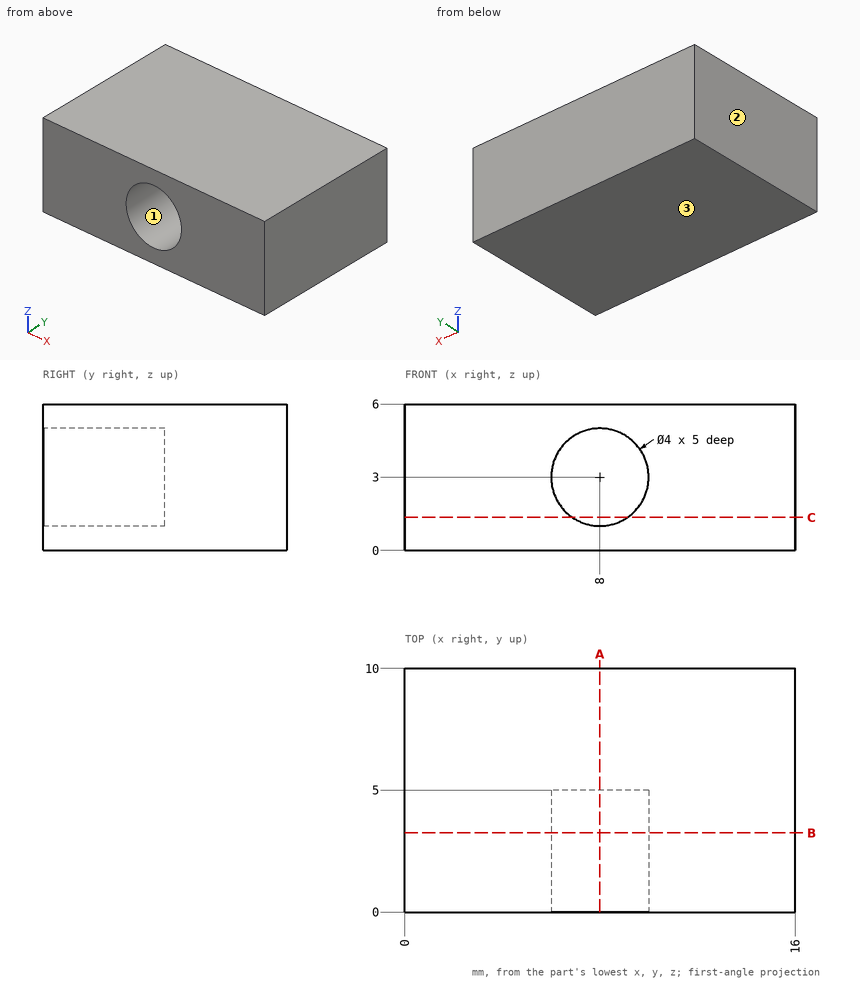
For this review, use the dimensioned drawing (mm, ordinates from the lowest corner) and the shaded views. Coordinates: 2 decimals unless noted, no trailing zeros. Loops run counter-clockwise (first coordinate to the right, second up) from the corner with the lowest first, then second, coordinate; pieces in that order, holes last.
1. For line 1 (X direction, y = 3.75, z = 3); line 2 (Z direction, x = 7.5, y = 4.5); line 3 (X direction, y = 3.75, z = 3.7), list the stretches that pass through material, from the lowest coordinate up.
2. Add section A-A, the plane x = 8. Give the boundary of the cut face in (y, z).
3. Add section C-C, the plane z = 1.35. Give the boundary of the cut face in (x, y), then the cut area to 3 significant figures.
4. Insertion check: P1, Ø1, axis at x = 13, y = 8, coming from the -Z side; P2, Ø1, axis at x = 8.5, z = 3.5, coming from the -Y side. Each pin has a flat end and moves straight along its axis. Give the tip position at first contact, or say it passes through.
5. Add section B-B, the plane y = 3.25. Give the boundary of the cut face in (x, z).
6. Mouldability with a two-part tool opening along Z and no side actions: class the marked faces 1, 2 and 3 as +Z half, -Z half, draft (parallel to the pull), parting line (faces both ways), or undercut.
Result:
1. line 1: x = 0 to 6, 10 to 16
1. line 2: z = 0 to 1.06, 4.94 to 6
1. line 3: x = 0 to 6.13, 9.87 to 16
2. outline: (0, 0) - (10, 0) - (10, 6) - (0, 6) - (0, 5) - (5, 5) - (5, 1) - (0, 1) - close
3. outline: (0, 0) - (6.87, 0) - (6.87, 5) - (9.13, 5) - (9.13, 0) - (16, 0) - (16, 10) - (0, 10) - close
3. area: 149 mm2
4. P1: stops at z = 0
4. P2: stops at y = 5
5. outline: (0, 0) - (16, 0) - (16, 6) - (0, 6) - close; hole circle Ø4 at (8, 3)
6. face 1: undercut
6. face 2: draft
6. face 3: -Z half
